Can you work these out from the model? Positions are in its coordinate system, mm. Face numbers are marked on the shaded views. A direction names the side the tool comes from. Give positions to 0.01 mm unless a question says otherwise; leave off trailing zeros. Order: outer loops, then holes, each group sorted by start corner. A loop starts at its lowest first (then second) coordinate and runs counter-clockwise, first axis right, second up. Notation, with made-up numbers: M 78.5,16 L 96.5,16 A20 ccw 96.5,52 Z; hole C -28.75,48.5 d9. An arc over 180 degrees is marked long. Write each question's results on one line, items separated by ' | '.
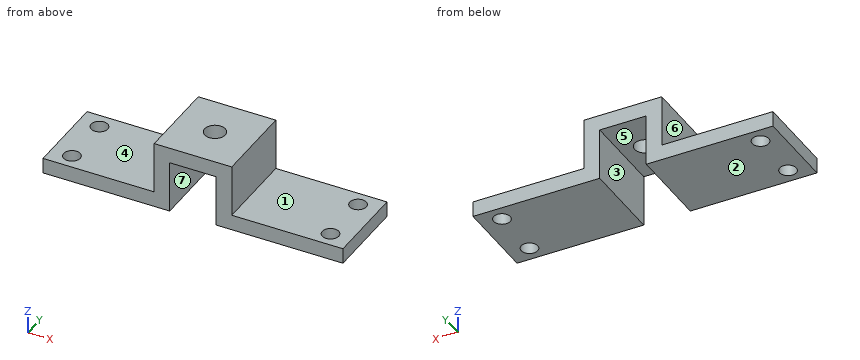
from build123d import *

# Parameters (mm, degrees)
EXTRUDE_1_DEPTH     = 16
SKETCH_2_R          = 2
SKETCH_2_R_2        = 1.59996579
CUT_EXTRUDE_1_DEPTH = 16


with BuildPart() as part:
    # 草图1 → 凸台-拉伸1 (new body)
    with BuildSketch(Plane(origin=(0, 0, 0), x_dir=(1, 0, 0), z_dir=(0, 1, 0))):
        Polygon((0, 0), (24.5, 0), (24.5, -10), (33.5, -10), (33.5, 0), (58, 0), (58, -3), (36.5, -3), (36.5, -13), (21.5, -13), (21.5, -3), (0, -3), align=None)
    extrude(amount=EXTRUDE_1_DEPTH)

    # 草图2 → 切除-拉伸1 (cut)
    with BuildSketch(Plane.XY.offset(13)):
        with Locations((29, 8)):
            Circle(SKETCH_2_R)
        with Locations((4, 13)):
            Circle(SKETCH_2_R_2)
        with Locations((4, 3)):
            Circle(SKETCH_2_R_2)
        with Locations((54, 13)):
            Circle(SKETCH_2_R_2)
        with Locations((54, 3)):
            Circle(SKETCH_2_R_2)
    extrude(amount=-CUT_EXTRUDE_1_DEPTH, mode=Mode.SUBTRACT)


solid = part.part
(1) For the marked faces 1, 2 and 3, which set-ups out of +Z, -Z, +X, -X, +Y, -Y let a thin tool reach every point of the face, with its end or its side?
Data:
face 1: +Z, +X, +Y, -Y | face 2: -Z, +X, -X, +Y, -Y | face 3: -Z, +Y, -Y
(2) I need wall thicknesses on L1, parallel to Y at x = 4, z = 0.8; L2, parallel to X at y = 14.5, z = 6; L3, parallel to X at y = 14, z = 0.5. Which ranges of each line are inside material? Lowest first, please. Write a range as from..to.
Data:
L1: y = 0..1.4, 4.6..11.4, 14.6..16 | L2: x = 21.5..24.5, 33.5..36.5 | L3: x = 0..2.75, 5.25..24.5, 33.5..52.75, 55.25..58
(3) Imagine slicing it at D-D, the plane y = 8. Write out the boundary of the cut face in (x, z).
Data:
outline: M 0,0 L 24.5,0 L 24.5,10 L 27,10 L 27,13 L 21.5,13 L 21.5,3 L 0,3 Z; M 31,10 L 33.5,10 L 33.5,0 L 58,0 L 58,3 L 36.5,3 L 36.5,13 L 31,13 Z
(4) Imagine slicing it at A-A, the plane x = 4. Write out the boundary of the cut face in (y, z).
Data:
outline: M 0,0 L 1.4,0 L 1.4,3 L 0,3 Z; M 4.6,0 L 11.4,0 L 11.4,3 L 4.6,3 Z; M 14.6,0 L 16,0 L 16,3 L 14.6,3 Z
(5) Will these pins go through, and if not, where does the flat tip stop? P1, Ø7, axis at x = 29, y = 11.5, coming from the -Z side; P2, Ø5, axis at y = 4, z = 10.5, coming from the -X side; P3, Ø5, axis at y = 4.5, z = 9.5, coming from the +X side.
Data:
P1: stops at z = 10 | P2: stops at x = 21.5 | P3: stops at x = 36.5
(6) We'd pull the mould along X, two halves only. Please class the marked faces 4, 5, 6 and 7: +X half, -X half, draft (parallel to the pull), parting line (faces both ways), or undercut.
Data:
face 4: draft | face 5: undercut | face 6: -X half | face 7: undercut
(7) Imagine slicing it at C-C, the plane z = 7.25. Write out the boundary of the cut face in (x, y).
Data:
outline: M 21.5,0 L 24.5,0 L 24.5,16 L 21.5,16 Z; M 33.5,0 L 36.5,0 L 36.5,16 L 33.5,16 Z
(8) Imagine slicing it at B-B, the plane y = 13. Write out the boundary of the cut face in (x, z).
Data:
outline: M 0,0 L 2.4,0 L 2.4,3 L 0,3 Z; M 5.6,0 L 24.5,0 L 24.5,10 L 33.5,10 L 33.5,0 L 52.4,0 L 52.4,3 L 36.5,3 L 36.5,13 L 21.5,13 L 21.5,3 L 5.6,3 Z; M 55.6,0 L 58,0 L 58,3 L 55.6,3 Z
